```python
from build123d import *

# Parameters (mm, degrees)
PAD002_DEPTH = 10
PAD001_DEPTH = 78
SKETCH_W     = 59
SKETCH_H     = 10
PAD_DEPTH    = 2
FILLET_R     = 2


with BuildPart() as pad002:
    # Sketch002 → Pad002 (new body)
    with BuildSketch(Plane.XZ):
        Polygon((8.152621, 6), (29.5, 34.945599), (50.847379, 6), align=None)
        Polygon((6, 13.189994), (25.772379, 40), (6, 66.810006), align=None)
        Polygon((8.152621, 74), (29.5, 45.054401), (50.847379, 74), align=None)
        Polygon((33.227621, 40), (53, 13.189994), (53, 66.810006), align=None)
    extrude(amount=PAD002_DEPTH)


with BuildPart() as pad001:
    # Sketch001 → Pad001 (new body)
    with BuildSketch(Plane.XY):
        Polygon((0, 0), (0, -8.6), (2.6, -8.6), (2.6, -7.5), (1.1, -7.5), (1.1, -5.5), (2.6, -5.5), (2.6, -1.5), (56.4, -1.5), (56.4, -5.5), (57.9, -5.5), (57.9, -7.5), (56.4, -7.5), (56.4, -8.6), (59, -8.6), (59, 0), align=None)
    extrude(amount=PAD001_DEPTH)


with BuildPart() as f_4_relay:
    # Sketch → Pad (new body)
    with BuildSketch(Plane.XY):
        with Locations((29.5, -5)):
            Rectangle(SKETCH_W, SKETCH_H)
    extrude(amount=PAD_DEPTH)

    # Fusion: union Pad001
    add(pad001.part)

    # Cut: cut Pad002
    add(pad002.part, mode=Mode.SUBTRACT)

    # Fillet
    fillet_edges = [f_4_relay.edges().sort_by_distance(p)[0] for p in [
        (53, -0.75, 13.189994),
        (25.772379, -0.75, 40),
        (50.847379, -0.75, 6),
        (33.227621, -0.75, 40),
        (53, -0.75, 66.810006),
        (6, -0.75, 66.810006),
        (50.847379, -0.75, 74),
        (29.5, -0.75, 45.054401),
        (29.5, -0.75, 34.945599),
        (8.152621, -0.75, 74),
        (8.152621, -0.75, 6),
        (6, -0.75, 13.189994),
    ]]
    fillet(fillet_edges, radius=FILLET_R)


solid = f_4_relay.part
```
Verification items for the finished model (mm, model axes). A direction names the side the tool comes from. Round coordinates to 2 decimals unless told otherwise and drop trailing zeros. Write each loop counter-clockwise with the first axis right and the second up, starting at its lowest first coordinate (ties: lowest second). Pieces come first, ordered by that corner, then holes.
1. Section check C-C on x = 50.5. Enter the section's corners in (y, z).
2. Access from +Z, -Z, +X, -X, +Y, -Y to the whole of each face (thin tool, end or side, straight path). Record for faces 1 (the flat face through (19.075, -0.74, 59.19)), 2 (the flat face through (27, -1, 78)), 3 (the flat face through (2.6, -4, 39)).
3. Section check A-A on z = 40. Enter the section's corners in (x, y).
4. Draft check along Y on faces 4 (the flat face through (30, -1, 74)), 5 (the flat face through (2, -7.5, 39)), 6 (the flat face through (29, -1.5, 39)), 7 (the flat face through (57, -7.5, 39)). Enter one of: +Y half, -Y half, draft (parallel to the pull), parting line (faces both ways), or undercut.
5. Section check B-B on x = 32. Enter the section's corners in (y, z), plus the area to 3 significant figures.
6. Gauge pin test, flat ends, axial feed: P1, Ø1.3, axis at x = 58, z = 43.5, coming from the -Y side; P2, Ø1.5, axis at x = 7.5, z = 22.5, coming from the +Y side; P3, Ø1.5, axis at x = 35.5, y = -2.5, coming from the +Z side; P4, Ø10, axis at x = 22.5, z = 17.5, coming from the -Y side. Record the tip position at first contact, or that the pin passes through.
7. Scan lines: L1, parallel to X at y = -3.5, z = 19.5; L2, parallel to X at y = -7.25, z = 13; L3, parallel to Z at x = 15, y = -7. Record each from-to range of solid material in increasing order.
8. Section check D-D on z = 26. Enter the section's corners in (x, y), plus the area to 3 significant figures.
Answer:
1. outline: (-10, 0) - (0, 0) - (0, 17.33) - (-1.5, 17.33) - (-1.5, 2) - (-10, 2) - close; (-1.5, 62.67) - (0, 62.67) - (0, 78) - (-1.5, 78) - close
2. face 1: +Y, -Y
2. face 2: +Z, +X, -X, +Y, -Y
2. face 3: +Z, -Y
3. outline: (0, -8.6) - (2.6, -8.6) - (2.6, -7.5) - (1.1, -7.5) - (1.1, -5.5) - (2.6, -5.5) - (2.6, -1.5) - (6, -1.5) - (6, 0) - (0, 0) - close; (25.29, -1.5) - (33.71, -1.5) - (33.71, 0) - (25.29, 0) - close; (53, -1.5) - (56.4, -1.5) - (56.4, -5.5) - (57.9, -5.5) - (57.9, -7.5) - (56.4, -7.5) - (56.4, -8.6) - (59, -8.6) - (59, 0) - (53, 0) - close
4. face 4: draft
4. face 5: undercut
4. face 6: -Y half
4. face 7: undercut
5. outline: (-10, 0) - (0, 0) - (0, 6) - (-1.5, 6) - (-1.5, 2) - (-10, 2) - close; (-1.5, 31.56) - (0, 31.56) - (0, 48.44) - (-1.5, 48.44) - close; (-1.5, 74) - (0, 74) - (0, 78) - (-1.5, 78) - close
5. area: 57.3 mm2
6. P1: stops at y = -8.6
6. P2: passes through
6. P3: stops at z = 2
6. P4: stops at y = -1.5
7. L1: x = 0 to 2.6, 56.4 to 59
7. L2: x = 0 to 1.1, 57.9 to 59
7. L3: z = 0 to 2
8. outline: (0, -8.6) - (2.6, -8.6) - (2.6, -7.5) - (1.1, -7.5) - (1.1, -5.5) - (2.6, -5.5) - (2.6, -1.5) - (6, -1.5) - (6, 0) - (0, 0) - close; (15.45, -1.5) - (22.9, -1.5) - (22.9, 0) - (15.45, 0) - close; (36.1, -1.5) - (43.55, -1.5) - (43.55, 0) - (36.1, 0) - close; (53, -1.5) - (56.4, -1.5) - (56.4, -5.5) - (57.9, -5.5) - (57.9, -7.5) - (56.4, -7.5) - (56.4, -8.6) - (59, -8.6) - (59, 0) - (53, 0) - close
8. area: 71.3 mm2
